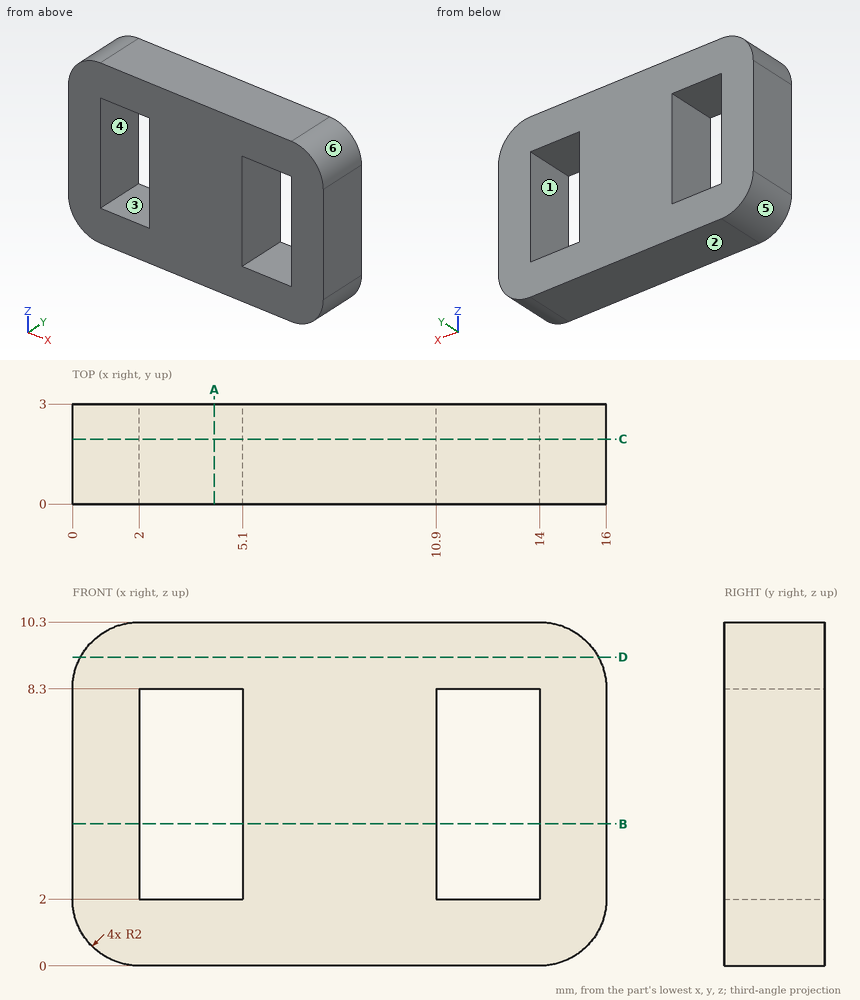
Geometry check sheet. Reference: drawing and pictorial views, mm from the part's lowest x, y, z. A direction names the side the tool comes from. Round coordinates to 2 decimals unless told otherwise and drop trailing zeros. Order: outer loops, then holes, each group sorted by start corner. A loop starts at its lowest first (then second) coordinate and runs counter-clockwise, first axis right, second up. Notation, with made-up numbers: (27.5, 78.5) -> (55.5, 78.5) arc R21 ccw to (55.5, 96.5) -> close; hole circle Ø1 at (50, 77.25). An arc over 180 degrees is marked (long way). One line per item, written item: value. Start each with the question number.
Q1. Cross-section at D-D (z = 9.25). Record the boundary of the cut face in (x, y), and give its area (3 significant figures).
Q2. Cross-section at B-B (z = 4.25). Record the boundary of the cut face in (x, y).
Q3. Cross-section at C-C (y = 1.95). Record the boundary of the cut face in (x, z), and give its area (3 significant figures).
Q4. Cross-section at A-A (x = 4.25). Record the boundary of the cut face in (y, z).
Q5. Mould release check, pull along Z, two halves, no side actions. Record for the marked faces 3, 4, 5 and 6: pulls with the +Z half, pulls with the -Z half, needs draft (parallel to the pull), parting line crosses it, or undercut.
Q6. Thickness scan on line 1 (X direction, y = 1.15, z = 6.75); line 2 (Z direction, x = 13.5, y = 1.55); line 3 (Z direction, x = 14.25, y = 0.75). Record the ranges inside material, lowest first.
Q7. Set-up check for the marked faces 1 and 2: record each of +Z, -Z, +X, -X, +Y, -Y from which the full face is reachable in a straight line by a thin tool's end or side.
Completed:
1. outline: (0.24, 0) -> (15.76, 0) -> (15.76, 3) -> (0.24, 3) -> close
1. area: 46.6 mm²
2. outline: (0, 0) -> (2, 0) -> (2, 3) -> (0, 3) -> close; (5.1, 0) -> (10.9, 0) -> (10.9, 3) -> (5.1, 3) -> close; (14, 0) -> (16, 0) -> (16, 3) -> (14, 3) -> close
3. outline: (0, 2) arc R2 ccw to (2, 0) -> (14, 0) arc R2 ccw to (16, 2) -> (16, 8.3) arc R2 ccw to (14, 10.3) -> (2, 10.3) arc R2 ccw to (0, 8.3) -> close; hole (2, 2) -> (5.1, 2) -> (5.1, 8.3) -> (2, 8.3) -> close; hole (10.9, 2) -> (14, 2) -> (14, 8.3) -> (10.9, 8.3) -> close
3. area: 122 mm²
4. outline: (0, 0) -> (3, 0) -> (3, 2) -> (0, 2) -> close; (0, 8.3) -> (3, 8.3) -> (3, 10.3) -> (0, 10.3) -> close
5. face 3: undercut
5. face 4: undercut
5. face 5: pulls with the -Z half
5. face 6: pulls with the +Z half
6. line 1: x = 0 to 2, 5.1 to 10.9, 14 to 16
6. line 2: z = 0 to 2, 8.3 to 10.3
6. line 3: z = 0.02 to 10.28
7. face 1: +Y, -Y
7. face 2: -Z, +X, -X, +Y, -Y
